from build123d import *

# Parameters (mm, degrees)
SKETCH1_R           = 22
SKETCH1_R_2         = 19
BOSS_EXTRUDE1_DEPTH = 6.5
SKETCH2_R           = 19
BOSS_EXTRUDE2_DEPTH = 4
CHAMFER1_SIZE       = 2.5
SKETCH3_R           = 3
CUT_EXTRUDE1_DEPTH  = 4
SKETCH5_R           = 8.5
BOSS_EXTRUDE3_DEPTH = 6.5
CHAMFER3_SIZE       = 2.5
SKETCH6_R           = 6
BOSS_EXTRUDE4_DEPTH = 10
FILLET2_R           = 1
SKETCH7_R           = 4
CUT_EXTRUDE2_DEPTH  = 23
SKETCH8_R           = 1.5
CUT_EXTRUDE3_DEPTH  = 6.5
FILLET3_R           = 1


with BuildPart() as part:
    # Sketch1 → Boss-Extrude1 (new, symmetric)
    with BuildSketch(Plane.XY):
        with Locations(Location((0, 0, 0), (0, 0, 180))):
            Circle(SKETCH1_R)
        with Locations(Location((0, 0, 0), (0, 0, 180))):
            Circle(SKETCH1_R_2, mode=Mode.SUBTRACT)
    extrude(amount=BOSS_EXTRUDE1_DEPTH, both=True)

    # Sketch2 → Boss-Extrude2 (add, symmetric)
    with BuildSketch(Plane.XY):
        with Locations(Location((0, 0, 0), (0, 0, 180))):
            Circle(SKETCH2_R)
    extrude(amount=BOSS_EXTRUDE2_DEPTH, both=True)

    # Chamfer1
    chamfer1_edges = [part.edges().sort_by_distance(p)[0] for p in [
        (19, 0, -4),
        (19, 0, 4),
    ]]
    chamfer(chamfer1_edges, length=CHAMFER1_SIZE - 0.0001)  # a hair under: the kernel refuses the full size

    # Sketch3 → Cut-Extrude1 (cut, symmetric)
    with BuildSketch(Plane.XY):
        with Locations((0, 12.5)):
            Circle(SKETCH3_R)
        with Locations((8.838834765, 8.838834765)):
            Circle(SKETCH3_R)
        with Locations((12.5, 0)):
            Circle(SKETCH3_R)
        with Locations((8.838834765, -8.838834765)):
            Circle(SKETCH3_R)
        with Locations((0, -12.5)):
            Circle(SKETCH3_R)
        with Locations((-8.838834765, -8.838834765)):
            Circle(SKETCH3_R)
        with Locations((-12.5, 0)):
            Circle(SKETCH3_R)
        with Locations((-8.838834765, 8.838834765)):
            Circle(SKETCH3_R)
    extrude(amount=CUT_EXTRUDE1_DEPTH, both=True, mode=Mode.SUBTRACT)

    # Sketch5 → Boss-Extrude3 (add, symmetric)
    with BuildSketch(Plane.XY):
        with Locations(Location((0, 0, 0), (0, 0, 180))):
            Circle(SKETCH5_R)
    extrude(amount=BOSS_EXTRUDE3_DEPTH, both=True)

    # Chamfer3
    chamfer3_edges = [part.edges().sort_by_distance(p)[0] for p in [
        (8.5, 0, -6.5),
        (8.5, 0, 6.5),
    ]]
    chamfer(chamfer3_edges, length=CHAMFER3_SIZE - 0.0001)  # a hair under: the kernel refuses the full size

    # Sketch6 → Boss-Extrude4 (add)
    with BuildSketch(Plane.XY.offset(6.5)):
        Circle(SKETCH6_R)
    extrude(amount=BOSS_EXTRUDE4_DEPTH)

    # Fillet2
    fillet2_edges = [part.edges().sort_by_distance(p)[0] for p in [
        (-6, 0, 16.5),
    ]]
    fillet(fillet2_edges, radius=FILLET2_R)

    # Sketch7 → Cut-Extrude2 (cut)
    with BuildSketch(Plane.XY.offset(16.5)):
        Circle(SKETCH7_R)
    extrude(amount=-CUT_EXTRUDE2_DEPTH, mode=Mode.SUBTRACT)

    # Sketch8 → Cut-Extrude3 (cut, symmetric)
    with BuildSketch(Plane(origin=(0, 0, 0), x_dir=(1, 0, 0), z_dir=(0, 1, 0))):
        with Locations(Location((0, -10.5, 0), (0, 0, 270))):
            Circle(SKETCH8_R)
    extrude(amount=CUT_EXTRUDE3_DEPTH, both=True, mode=Mode.SUBTRACT)

    # Fillet3
    fillet3_edges = [part.edges().sort_by_distance(p)[0] for p in [
        (22, 0, -6.5),
        (22, 0, 6.5),
    ]]
    fillet(fillet3_edges, radius=FILLET3_R)


solid = part.part
The listing builds one solid part. Answer for the finished solid, in the listing's coordinates (mm). A direction names the side the tool comes from. Round coordinates to 2 decimals unless told otherwise and drop trailing zeros. Order: outer loops, then holes, each group sorted by start corner. A loop starts at its lowest first (then second) coordinate and runs counter-clockwise, first axis right, second up. Notation, with made-up numbers: (1.25, 74.25) -> (18.25, 74.25) arc R19 cw to (18.25, 94.25) -> close; hole circle Ø9 at (28.25, 77.25). An arc over 180 degrees is marked (long way). Write each question's results on one line, items separated by ' | '. Start each with the question number.
Q1. Find section B-B (z = 10.5). Determine the outline of the cut face in (x, y), then the cut area to 3 significant figures.
Q2. Straight lines are drawn through the part: probe 1 along X at (y, z) = (11, -3.25); probe 2 along Y at (x, z) = (-0.5, 4.75); probe 3 along X at (y, z) = (8, 0). For each, find the intervals that lie inside material, in ascending order. Write a range as from..to.
Q3. Find section A-A (x = 0). Give the number of separate pieces and of enclosed holes in the cut face, then the cut area to 3 significant figures.
Q4. Which of the six approach directions +Z, -Z, +X, -X, +Y, -Y give full straight-line access (tool end or side, diameter ignored) to faces 1 (the flat face through (5, 7.3, 4)), 2 (the flat face through (5, 7.3, -4)), 3 (the cylindrical face through (11.7, 9.74, -0.06))?
Q5. The mould has two halves that part along Z. Classify faces 4 (the cylindrical face through (3.695, -1.532, 5.161)), 5 (the conical face through (6.116, -0.269, 6.379)), 6 (the cylindrical face through (0, 5, 9)): pulls with the +Z half, pulls with the -Z half, needs draft (parallel to the pull), parting line crosses it, or undercut.
Q6. Each of these flat-tipped pins is pushed along its axis until it touches: pin 1 (21 mm diameter, centred on x = 4, y = 5, fed in from +Z); pin 2 (5.5 mm diameter, centred on x = 8.84, y = -8.84, fed in from -Z); pin 3 (2 mm diameter, centred on x = 4, z = 3, fed in from +Y); pin 4 (9.5 mm diameter, centred on x = 12.5, y = 0, fed in from -Z). Where does it stop, or does it pass through?
Worked answers:
1) outline: (-1.5, -5.81) -> (-1.5, -3.71) arc R4 cw to (-1.5, 3.71) -> (-1.5, 5.81) arc R6 ccw to start; (1.5, -5.81) arc R6 ccw to (1.5, 5.81) -> (1.5, 3.71) arc R4 cw to (1.5, -3.71) -> close | area: 50.6 mm2
2) probe 1: x = -19.05..-10.92, -6.76..-2.6, 2.6..6.76, 10.92..19.05 | probe 2: y = -21.99..-17.24, -7.73..-3.97, 3.97..7.73, 17.24..21.99 | probe 3: x = -20.49..-11.72, -5.96..5.96, 11.72..20.49
3) separate pieces: 6 | enclosed holes: 0 | area: 294 mm2
4) face 1: +Z | face 2: -Z | face 3: +Z, -Z
5) face 4: needs draft | face 5: pulls with the +Z half | face 6: undercut
6) pin 1: stops at z = 16.5 | pin 2: passes through | pin 3: stops at y = 21.79 | pin 4: stops at z = -4.75
